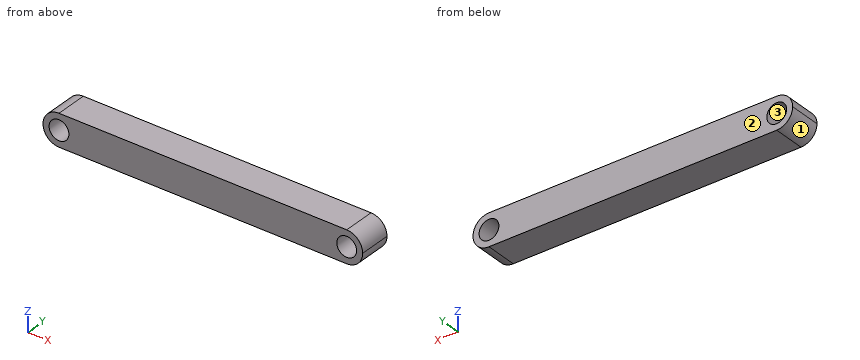
from build123d import *

# Parameters (mm, degrees)
F0_W     = 50
F0_H     = 5
F1_DEPTH = 2.5
F2_R     = 2.49999
F3_R     = 1.55
F4_DEPTH = 12.5


# Not quite as in the source:
# - a fillet or chamfer is up to 0.001 mm smaller than in the source, because OpenCascade refuses the exact size


with BuildPart() as f1:
    # F0 (on Front) → F1 (new body, symmetric)
    with BuildSketch(Plane.XZ):
        Rectangle(F0_W, F0_H)
    extrude(amount=F1_DEPTH, both=True)

    # F2 (radius 2.5 in the source; OpenCascade refuses exactly that, so slightly less here)
    f2_edges = [f1.edges().sort_by_distance(p)[0] for p in [
        (25, 0, 2.5),
        (25, 0, -2.5),
        (-25, 0, 2.5),
        (-25, 0, -2.5),
    ]]
    fillet(f2_edges, radius=F2_R)

    # F3 (on face) → F4 (cut, symmetric)
    with BuildSketch(Plane(origin=(0, 2.5, 0), x_dir=(-1, 0, 0), z_dir=(0, 1, 0))):
        with Locations((-22.5, 0)):
            Circle(F3_R)
        with Locations((22.5, 0)):
            Circle(F3_R)
    extrude(amount=F4_DEPTH, both=True, mode=Mode.SUBTRACT)


solid = f1.part
Work out the finished part from the listing and answer in its coordinate system (mm). Face numbers are marked on the shaded views. Give positions to 0.01 mm unless a question says otherwise; leave off trailing zeros. Order: outer loops, then holes, each group sorted by start corner. A loop starts at its lowest first (then second) coordinate and runs counter-clockwise, first axis right, second up. Notation, with made-up numbers: (-15.75, 77.25) -> (40.25, 77.25) arc R10 ccw to (40.25, 94.25) -> close; hole circle Ø11 at (-2, 35). An arc over 180 degrees is marked (long way). Answer as a JSON object with one key per item and string values. Group by question number.
1. Section B-B on x = -21.5 is taken. Determine the outline of the cut face in (y, z), plus the area to 3 significant figures.
2. A flat-ended cylindrical pin translates along its axis: pin 1 Ø2 at (y, z) = (-0.5, 1.5) entering from -X. Find the tip coordinate at first contact, or state that the pin passes through.
3. Section A-A on y = 0.95 is taken. Count the separate pieces of the cut face and the enclosed holes in it, plus the area to 3 significant figures.
4. The mould has two halves that part along X. Classify the marked faces 1, 2 and 3: released by +X, released by -X, zero draft, split by the parting line, or undercut.
5. Consider line 1 along Z through (x, y) = (22.5, -0.65); line 2 along X through (y, z) = (0.3, 1.3); line 3 along X through (y, z) = (-1.2, -1). Determine where each line is inside the solid, lowest interval first. Write a range as [from, to].
6. Section C-C on z = 0.45 is taken. Determine the outline of the cut face in (x, y).
Result sheet:
{
 "1": {"outline": "(-2.5, -2.5) -> (2.5, -2.5) -> (2.5, -1.18) -> (-2.5, -1.18) -> close; (-2.5, 1.18) -> (2.5, 1.18) -> (2.5, 2.5) -> (-2.5, 2.5) -> close", "area": "13.2 mm^2"},
 "2": {"pin 1": "stops at x = -24.95"},
 "3": {"separate pieces": "1", "enclosed holes": "2", "area": "230 mm^2"},
 "4": {"face 1": "released by -X", "face 2": "zero draft", "face 3": "undercut"},
 "5": {"line 1": "z = [-2.5, -1.55], [1.55, 2.5]", "line 2": "x = [-24.64, -23.34], [-21.66, 21.66], [23.34, 24.64]", "line 3": "x = [-24.79, -23.68], [-21.32, 21.32], [23.68, 24.79]"},
 "6": {"outline": "(-24.96, -2.5) -> (-23.98, -2.5) -> (-23.98, 2.5) -> (-24.96, 2.5) -> close; (-21.02, -2.5) -> (21.02, -2.5) -> (21.02, 2.5) -> (-21.02, 2.5) -> close; (23.98, -2.5) -> (24.96, -2.5) -> (24.96, 2.5) -> (23.98, 2.5) -> close"}
}
